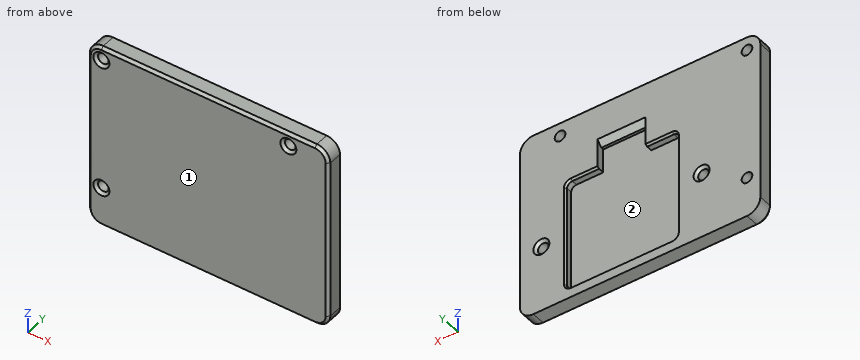
```python
from build123d import *

# Parameters (mm, degrees)
SKETCH_1_W          = 90
SKETCH_1_H          = 70
SKETCH_1_R          = 2
EXTRUDE_1_DEPTH     = 6
FILLET_1_R          = 5
SKETCH_2_W          = 42
SKETCH_2_H          = 42
CUT_EXTRUDE_1_DEPTH = 3
SKETCH_3_W          = 18
SKETCH_3_H          = 18
CUT_EXTRUDE_2_DEPTH = 3
FILLET_2_R          = 2
CHAMFER_1_SIZE      = 2
SKETCH_4_R          = 2
CUT_EXTRUDE_3_DEPTH = 5
CHAMFER_2_SIZE      = 1
CHAMFER_3_SIZE      = 1
CHAMFER_4_SIZE      = 0.5
CHAMFER_4_SIZE2     = 0.866025404


with BuildPart() as part:
    # Эскиз1 → Бобышка-Вытянуть1 (new body)
    # profile 1 of 2: a face of its own
    with BuildSketch(Plane(origin=(0, 0, 0), x_dir=(1, 0, 0), z_dir=(0, 1, 0))):
        with Locations((5, 5)):
            Rectangle(SKETCH_1_W, SKETCH_1_H)
        with Locations(Location((35, -25, 0), (0, 0, 270))):
            Circle(SKETCH_1_R, mode=Mode.SUBTRACT)
        with Locations(Location((-35, -25, 0), (0, 0, 270))):
            Circle(SKETCH_1_R, mode=Mode.SUBTRACT)
        with Locations((35, 25)):
            Circle(SKETCH_1_R, mode=Mode.SUBTRACT)
        with Locations(Location((-35, 25, 0), (0, 0, 270))):
            Circle(SKETCH_1_R, mode=Mode.SUBTRACT)
    # profile 2 of 2: a face of its own
    with BuildSketch(Plane(origin=(0, 0, 0), x_dir=(1, 0, 0), z_dir=(0, 1, 0))):
        with Locations((35, 25)):
            Circle(SKETCH_1_R)
    extrude(amount=EXTRUDE_1_DEPTH)

    # Скругление1
    fillet_1_edges = [part.edges().sort_by_distance(p)[0] for p in [
        (-40, 3, 30),
        (-40, 3, -40),
        (50, 3, -40),
        (50, 3, 30),
    ]]
    fillet(fillet_1_edges, radius=FILLET_1_R)

    # Эскиз2 → Вырез-Вытянуть1 (cut)
    with BuildSketch(Plane(origin=(0, 6, 0), x_dir=(1, 0, 0), z_dir=(0, 1, 0))):
        with Locations((12, 15)):
            Rectangle(SKETCH_2_W, SKETCH_2_H)
    extrude(amount=-CUT_EXTRUDE_1_DEPTH, mode=Mode.SUBTRACT)

    # Эскиз3 → Вырез-Вытянуть2 (cut)
    with BuildSketch(Plane(origin=(0, 6, 0), x_dir=(1, 0, 0), z_dir=(0, 1, 0))):
        with Locations((12, -6)):
            Rectangle(SKETCH_3_W, SKETCH_3_H)
    extrude(amount=-CUT_EXTRUDE_2_DEPTH, mode=Mode.SUBTRACT)

    # Скругление2
    fillet_2_edges = [part.edges().sort_by_distance(p)[0] for p in [
        (33, 4.5, -36),
        (33, 4.5, 6),
        (-9, 4.5, 6),
        (-9, 4.5, -36),
    ]]
    fillet(fillet_2_edges, radius=FILLET_2_R)

    # Фаска1
    chamfer_1_edges = [part.edges().sort_by_distance(p)[0] for p in [
        (12, 6, 15),
    ]]
    chamfer(chamfer_1_edges, length=CHAMFER_1_SIZE)

    # Эскиз4 → Вырез-Вытянуть3 (cut)
    with BuildSketch(Plane(origin=(0, 6, 0), x_dir=(1, 0, 0), z_dir=(0, 1, 0))):
        with Locations(Location((-18, 15, 0), (0, 0, 270))):
            Circle(SKETCH_4_R)
        with Locations(Location((42, 15, 0), (0, 0, 90))):
            Circle(SKETCH_4_R)
    extrude(amount=-CUT_EXTRUDE_3_DEPTH, mode=Mode.SUBTRACT)

    # Фаска2
    chamfer_2_edges = [part.edges().sort_by_distance(p)[0] for p in [
        (-18, 6, -17),
        (42, 6, -13),
    ]]
    chamfer(chamfer_2_edges, length=CHAMFER_2_SIZE)

    # Фаска3
    chamfer_3_edges = [part.edges().sort_by_distance(p)[0] for p in [
        (-35, 0, -27),
        (-35, 0, 23),
        (35, 0, 23),
        (-40, 0, -5),
        (5, 0, 30),
        (5, 0, -40),
        (50, 0, -5),
        (-38.535533906, 0, 28.535533906),
        (48.535533906, 0, 28.535533906),
        (48.535533906, 0, -38.535533906),
        (-38.535533906, 0, -38.535533906),
    ]]
    chamfer(chamfer_3_edges, length=CHAMFER_3_SIZE)

    # Фаска4
    chamfer_4_edges = [part.edges().sort_by_distance(p)[0] for p in [
        (26, 6, 6),
        (33, 6, -15),
        (-2, 6, 6),
        (-9, 6, -15),
        (12, 6, -36),
        (32.414213562, 6, 5.414213562),
        (-8.414213562, 6, 5.414213562),
        (-8.414213562, 6, -35.414213562),
        (32.414213562, 6, -35.414213562),
    ]]
    chamfer_4_side = [part.faces().sort_by_distance(p)[0] for p in [
        (-18, 6, -19.140175425),
    ]]
    chamfer(chamfer_4_edges, length=CHAMFER_4_SIZE, length2=CHAMFER_4_SIZE2, reference=chamfer_4_side[0])


solid = part.part
```
CAD build for the part. Positions are in the model's coordinates, mm. Face numbers are marked on the shaded views. Coordinates: 2 decimals unless noted, no trailing zeros. Order: outer loops, then holes, each group sorted by start corner. A loop starts at its lowest first (then second) coordinate and runs counter-clockwise, first axis right, second up.
(1) Saw through at D-D, the plane z = -15. Write the cut outline in (x, y).
Solution:
outline: (-40, 1) - (-39, 0) - (49, 0) - (50, 1) - (50, 6) - (45, 6) - (44, 5) - (44, 1) - (40, 1) - (40, 5) - (39, 6) - (33.5, 6) - (33, 5.13) - (33, 3) - (-9, 3) - (-9, 5.13) - (-9.5, 6) - (-15, 6) - (-16, 5) - (-16, 1) - (-20, 1) - (-20, 5) - (-21, 6) - (-40, 6) - close
(2) Saw through at B-B, the plane x = 35. Write the cut outline in (y, z).
Solution:
outline: (0, -39) - (1, -40) - (6, -40) - (6, 23) - (1, 23) - (0, 22) - close; (0, 28) - (1, 27) - (6, 27) - (6, 30) - (1, 30) - (0, 29) - close
(3) Mould opens along X. For the marked faces 1 and 2 say: released by +X, released by -X, zero draft, split by the parting line, or undercut.
Solution:
face 1: zero draft
face 2: undercut
(4) Saw through at C-C, the plane x = -3. Write the cut outline in (y, z).
Solution:
outline: (0, -39) - (1, -40) - (6, -40) - (6, -36.5) - (5.13, -36) - (3, -36) - (3, 6) - (5.13, 6) - (6, 6.5) - (6, 30) - (1, 30) - (0, 29) - close
(5) Saw through at A-A, the plane z = -25. Write the cut outline in (x, y), and give its area (3 significant figures).
Solution:
outline: (-40, 1) - (-39, 0) - (-38, 0) - (-37, 1) - (-37, 6) - (-40, 6) - close; (-33, 1) - (-32, 0) - (49, 0) - (50, 1) - (50, 6) - (33.5, 6) - (33, 5.13) - (33, 3) - (-9, 3) - (-9, 5.13) - (-9.5, 6) - (-33, 6) - close
area: 388 mm2
(6) Drill centre lines: L1, parallel to X at y = 3.5, z = -25; L2, parallel to X at y = 2.25, z = -15; L3, parallel to X at y = 3.5, z = -15. Where is each one in solid material? Low to high.
Solution:
L1: x = -40 to -37, -33 to -9, 33 to 50
L2: x = -40 to -20, -16 to 40, 44 to 50
L3: x = -40 to -20, -16 to -9, 33 to 40, 44 to 50
(7) Pin check, flat tips, straight feed: pin 1 Ø2 at (x, z) = (3, 22.5) entering from -Y; pin 2 Ø3 at (x, z) = (-17.5, -14.5) entering from +Y; pin 3 Ø3.5 at (x, z) = (-18, -15) entering from +Y. Stop position of each tip, or through.
Solution:
pin 1: stops at y = 0
pin 2: stops at y = 5.21
pin 3: stops at y = 1
